from build123d import *

# Parameters (mm, degrees)
SKETCH1_W           = 4
SKETCH1_H           = 6.6
BOSS_EXTRUDE1_REACH = 63.704
SKETCH21_R          = 4
BOSS_EXTRUDE2_REACH = 77.825
SKETCH22_R          = 4
CUT_EXTRUDE3_DEPTH  = 6.6
CUT_EXTRUDE4_DEPTH  = 6.6
CUT_EXTRUDE5_DEPTH  = 6.6
CHAMFER2_SIZE       = 0.25


with BuildPart() as part:
    # Sketch1 → Revolve-Thin1 (revolve)
    with BuildSketch(Plane(origin=(0, 0, 0), x_dir=(1, 0, 0), z_dir=(0, 1, 0))):
        with Locations((-2, 20.8)):
            Rectangle(SKETCH1_W, SKETCH1_H)
    revolve(axis=Axis((0, 0, -17.5), (0, 0, -1)))

    # Sketch21 → Boss-Extrude1 (add, up to next)
    with BuildSketch(Plane(origin=(-36.020185124, 0, -65.949410445), x_dir=(0.877628145, 0, -0.47934209), z_dir=(0.47934209, 0, 0.877628145)), mode=Mode.PRIVATE) as boss_extrude1_sk1:
        with Locations((9.970315475, 0)):
            Circle(SKETCH21_R)
    boss_extrude1_tool1 = extrude(boss_extrude1_sk1.sketch, amount=BOSS_EXTRUDE1_REACH, mode=Mode.PRIVATE) - part.part
    add(boss_extrude1_tool1.solids().sort_by_distance((-27.269956, 0, -70.728602))[0])

    # Sketch22 → Boss-Extrude2 (add, up to next)
    with BuildSketch(Plane(origin=(36.540728539, 0, -67.204649662), x_dir=(0.878534203, 0, 0.477679446), z_dir=(-0.477679446, 0, 0.878534203)), mode=Mode.PRIVATE) as boss_extrude2_sk1:
        with Locations((-9.935732483, 0)):
            Circle(SKETCH22_R)
    boss_extrude2_tool1 = extrude(boss_extrude2_sk1.sketch, amount=BOSS_EXTRUDE2_REACH, mode=Mode.PRIVATE) - part.part
    add(boss_extrude2_tool1.solids().sort_by_distance((27.811848, 0, -71.950745))[0])

    # Sketch29 → Cut-Extrude3 (cut)
    with BuildSketch(Plane(origin=(-36.020185124, 0, -65.949410445), x_dir=(-0.877628145, 0, 0.47934209), z_dir=(-0.47934209, 0, -0.877628145))):
        Polygon((-7.031266698, 1.20221696), (-9.541941515, 3.146399384), (-12.480990292, 1.944182424), (-12.909364252, -1.20221696), (-10.398689436, -3.146399384), (-7.459640658, -1.944182424), align=None)
    extrude(amount=-CUT_EXTRUDE3_DEPTH, mode=Mode.SUBTRACT)

    # Sketch30 → Cut-Extrude4 (cut)
    with BuildSketch(Plane(origin=(36.540728539, 0, -67.204649662), x_dir=(-0.878534203, 0, -0.477679446), z_dir=(0.477679446, 0, -0.878534203))):
        Polygon((12.87478126, 1.20221696), (10.364106444, 3.146399384), (7.425057666, 1.944182424), (6.996683706, -1.20221696), (9.507358523, -3.146399384), (12.4464073, -1.944182424), align=None)
    extrude(amount=-CUT_EXTRUDE4_DEPTH, mode=Mode.SUBTRACT)

    # Sketch18 → Cut-Extrude5 (cut)
    with BuildSketch(Plane.XY.offset(-17.5)):
        Polygon((1.58771324, 2.75), (-1.58771324, 2.75), (-3.175426481, 0), (-1.58771324, -2.75), (1.58771324, -2.75), (3.175426481, 0), align=None)
    extrude(amount=-CUT_EXTRUDE5_DEPTH, mode=Mode.SUBTRACT)

    # Chamfer2
    chamfer2_edges = [part.edges().sort_by_distance(p)[0] for p in [
        (-29.661371054, -0.370982732, -69.422461356),
        (-28.747628135, 2.174308172, -69.921528578),
        (-26.356212732, 2.545290904, -71.227669527),
        (-24.878540246, 0.370982732, -72.034743254),
        (-25.792283165, -2.174308172, -71.535676032),
        (-28.183698569, -2.545290904, -70.229535082),
        (25.417963429, -0.370982732, -73.252355328),
        (26.332649691, 2.174308172, -72.755019168),
        (28.726533979, 2.545290904, -71.453408693),
        (30.205732005, 0.370982732, -70.649134379),
        (29.291045743, -2.174308172, -71.146470539),
        (26.897161455, -2.545290904, -72.448081013),
        (2.38156986, 1.375, -17.5),
        (0, 2.75, -17.5),
        (-2.38156986, 1.375, -17.5),
        (-2.38156986, -1.375, -17.5),
        (0, -2.75, -17.5),
        (2.38156986, -1.375, -17.5),
    ]]
    chamfer(chamfer2_edges, length=CHAMFER2_SIZE)


solid = part.part
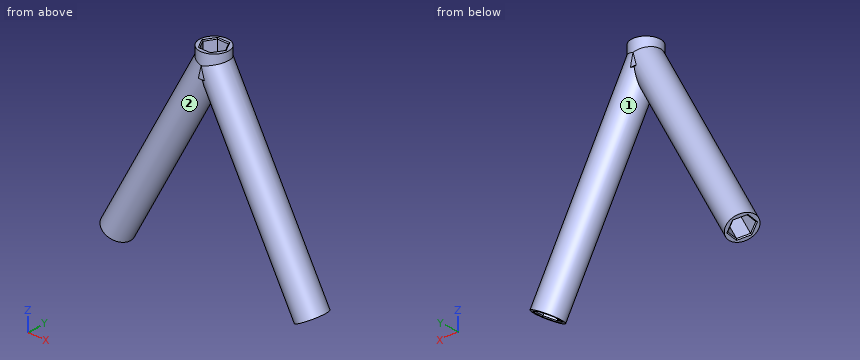
Here's how the part is built. I have some questions about the finished solid (model axes, mm). Face numbers are marked on the shaded views. Give positions to 0.01 mm unless a question says otherwise; leave off trailing zeros. Answer as a JSON object with one key per item and string values. Group by question number.
Item 1: I need wall thicknesses on L1, parallel to X at y = -1.25, z = -69; L2, parallel to X at y = 0, z = -40; L3, parallel to Z at x = -22.5, y = 1.5. Which ranges of each line are inside material? Lowest first, please.
Item 2: Thinking about a two-plate mould opening in X: for the marked faces 1 and 2, which applies, pulls with the +X half, pulls with the -X half, needs draft (parallel to the pull), parting line crosses it, or undercut?
Item 3: Will these pins go through, and if not, where does the flat tip stop? pin 1 (1 mm diameter, centred on x = -21, y = 0.5, fed in from +Z); pin 2 (3 mm diameter, centred on y = -3, z = -41, fed in from -X); pin 3 (3 mm diameter, centred on x = 0, y = 1, fed in from +Z).
Answer list:
{
 "1": {"L1": "x = -30.43 to -29.29, -23.05 to -22, 21.88 to 23.24, 29.48 to 30.53", "L2": "x = -15.04 to -5.93, 5.89 to 14.99", "L3": "z = -69.73 to -67.36, -65.81 to -54.26"},
 "2": {"face 1": "undercut", "face 2": "undercut"},
 "3": {"pin 1": "stops at z = -50.05", "pin 2": "stops at x = -15.6", "pin 3": "stops at z = -24.1"}
}
